Input: part model. Units: mm. Frame: model coordinates. Face numbers are marked on the shaded views. A direction names the side the tool comes from. Give positions to 0.01 mm unless a question says otherwise; leave off trailing zeros. Order: outer loops, then holes, each group sorted by start corner. A loop starts at its lowest first (then second) coordinate and runs counter-clockwise, first axis right, second up. Notation, with made-up numbers: M -20.75,64.5 L 7.25,64.5 A19 cw 7.25,97.5 Z; hole C 14.5,-10 d3. An arc over 180 degrees is marked long. Use a Markdown table: item, result.
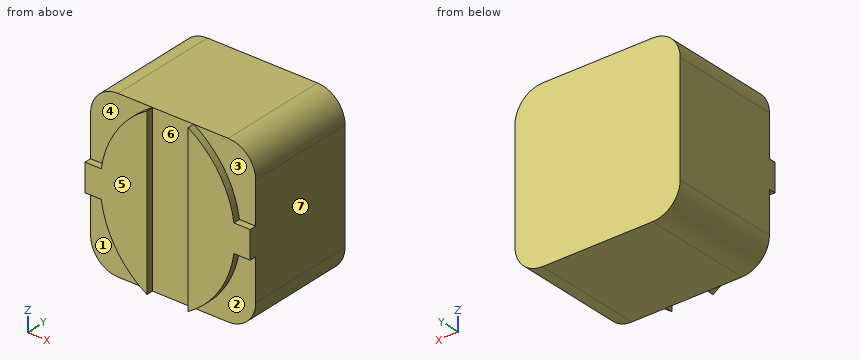
from build123d import *

# Parameters (mm, degrees)
SKETCH_2_W      = 12
SKETCH_2_H      = 12
EXTRUDE_1_DEPTH = 8
FILLET_1_R      = 2
EXTRUDE_START   = -0.5
EXTRUDE_2_DEPTH = 0.5
SKETCH_4_W      = 2
SKETCH_4_H      = 2
EXTRUDE_3_DEPTH = 0.5


# Read off the part's stored shape, not the designer's step: Бобышка-Вытянуть2
with BuildPart() as part:
    # Эскиз2 → Бобышка-Вытянуть1 (new body)
    with BuildSketch(Plane(origin=(0, 0, 0), x_dir=(1, 0, 0), z_dir=(0, 1, 0))):
        Rectangle(SKETCH_2_W, SKETCH_2_H)
    extrude(amount=EXTRUDE_1_DEPTH)

    # Скругление1
    fillet_1_edges = [part.edges().sort_by_distance(p)[0] for p in [
        (-6, 4, -6),
        (6, 4, -6),
        (6, 4, 6),
        (-6, 4, 6),
    ]]
    fillet(fillet_1_edges, radius=FILLET_1_R)

    # Бобышка-Вытянуть2 outline → Бобышка-Вытянуть2 (add)
    with BuildSketch(Plane(origin=(0, 0, 0), x_dir=(1, 0, 0), z_dir=(0, 1, 0)).offset(EXTRUDE_START)):
        with BuildLine():
            Line((-1.5, -6), (-1.5, 6))
            ThreePointArc((-1.5, 6), (-4.894448725, 0), (-1.5, -6))
        make_face()
        with BuildLine():
            Line((1.5, 6), (1.5, -6))
            ThreePointArc((1.5, -6), (4.894448725, 0), (1.5, 6))
        make_face()
    extrude(amount=EXTRUDE_2_DEPTH)

    # Эскиз4 → Бобышка-Вытянуть3 (add)
    with BuildSketch(Plane.XZ):
        with Locations((-5, 0)):
            Rectangle(SKETCH_4_W, SKETCH_4_H)
        with Locations((5, 0)):
            Rectangle(SKETCH_4_W, SKETCH_4_H)
    extrude(amount=EXTRUDE_3_DEPTH)


solid = part.part
1) Cut plane D-D on z = 4.5. Return loops of the section in (x, y), and give its area (3 significant figures).
Response values:
| item | result |
|---|---|
| outline | M -5.94,0 L -3.26,0 L -3.26,-0.5 L -1.5,-0.5 L -1.5,0 L 1.5,0 L 1.5,-0.5 L 3.26,-0.5 L 3.26,0 L 5.94,0 L 5.94,8 L -5.94,8 Z |
| area | 96.7 mm² |
2) Mould query, pull axis X, two halves, no side actions, for the marked faces 5, 6 and 7. Classes: released by +X, released by -X, zero draft, split by the parting line, or undercut.
Response values:
| item | result |
|---|---|
| face 5 | zero draft |
| face 6 | undercut |
| face 7 | released by +X |
3) Cut plane B-B on z = 2.25. Return loops of the section in (x, y).
Response values:
| item | result |
|---|---|
| outline | M -6,0 L -4.52,0 L -4.52,-0.5 L -1.5,-0.5 L -1.5,0 L 1.5,0 L 1.5,-0.5 L 4.52,-0.5 L 4.52,0 L 6,0 L 6,8 L -6,8 Z |
4) Material intervals for line 1 (Y direction, x = 0, z = 4.5); line 2 (Z direction, x = -5.5, y = 2); line 3 (X direction, y = 4, z = 5), sorted ascending. Write a range as from..to.
Response values:
| item | result |
|---|---|
| line 1 | y = 0..8 |
| line 2 | z = -5.32..5.32 |
| line 3 | x = -5.73..5.73 |
5) Cut plane A-A on y = 6.5. Return loops of the section in (x, z), and give its area (3 significant figures).
Response values:
| item | result |
|---|---|
| outline | M -6,-4 A2 ccw -4,-6 L 4,-6 A2 ccw 6,-4 L 6,4 A2 ccw 4,6 L -4,6 A2 ccw -6,4 Z |
| area | 141 mm² |
6) First-contact query: pin 1 Ø0.9 at (x, z) = (0.5, -3) entering from -Y. Flat tip, straight axial feed; report the tip coordinate or a pass-through.
Response values:
| item | result |
|---|---|
| pin 1 | stops at y = 0 |
7) Reachability of the marked faces 1, 2, 3 and 4 from +Z, -Z, +X, -X, +Y, -Y: full face, straight path, thin tool, end or side. Return the list, or none.
Response values:
| item | result |
|---|---|
| face 1 | -Z, -X, -Y |
| face 2 | -Z, +X, -Y |
| face 3 | +Z, +X, -Y |
| face 4 | +Z, -X, -Y |
8) Cut plane C-C on x = -3.5. Return loops of the section in (y, z).
Response values:
| item | result |
|---|---|
| outline | M -0.5,-4.19 L 0,-4.19 L 0,-6 L 8,-6 L 8,6 L 0,6 L 0,4.19 L -0.5,4.19 Z |
